Part model, mm, in its own coordinate system. Coordinates: 2 decimals unless noted, no trailing zeros. Order: outer loops, then holes, each group sorted by start corner. A loop starts at its lowest first (then second) coordinate and runs counter-clockwise, first axis right, second up.
1) Cut at B-B (x = -22.5). List the corners of the cut face in (y, z).
2) Wall check: L1, parallel to X at y = 2.5, z = 0.3; L2, parallel to Y at x = -64, z = 0.4; L3, parallel to X at y = -26, z = 0.2. Give the ranges that are in metal, low to high.
3) Pin check, flat tips, straight feed: pin 1 Ø0.9 at (x, z) = (-85, 1) entering from -Y; pin 2 Ø10 at (x, y) = (-76.5, -68.5) entering from -Z; pin 3 Ø1 at (y, z) = (41.5, 1.5) entering from -X; pin 4 Ø1.5 at (x, z) = (-86.5, 2) entering from +Y. Stop position of each tip, or through.
4) Cut at A-A (y = -1.5). List the corners of the cut face in (x, z), and give its area (3 significant figures).
5) Cut at C-C (z = 0.45). Give the number of separate pieces and of enclosed holes in the cut face, and give its area (3 significant figures).
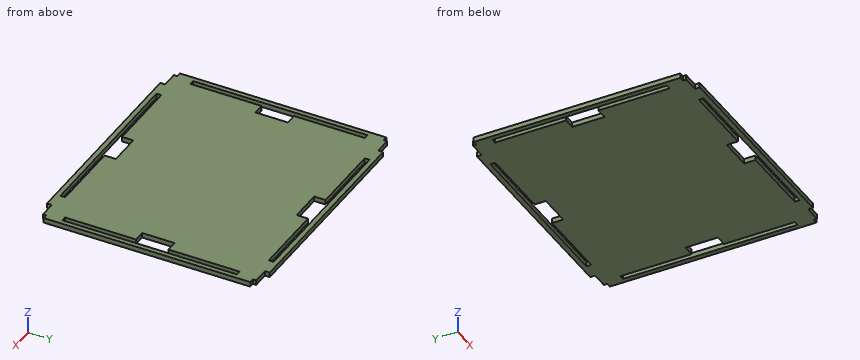
```python
from build123d import *

# Parameters (mm, degrees)
BOSS_EXTRUDE1_DEPTH = 3


with BuildPart() as part:
    # Sketch1 → Boss-Extrude1 (new body)
    with BuildSketch(Plane.XY):
        Polygon((46.640816327, 44.833717619), (-83.359183673, 44.833717619), (-83.359183673, 41.833717619), (-93.359183673, 41.833717619), (-93.359183673, 39.833717619), (-96.359183673, 39.833717619), (-96.359183673, -88.166282381), (-93.359183673, -88.166282381), (-93.359183673, -90.166282381), (-83.359183673, -90.166282381), (-83.359183673, -93.166282381), (46.640816327, -93.166282381), (46.640816327, -90.166282381), (56.640816327, -90.166282381), (56.640816327, -88.166282381), (59.640816327, -88.166282381), (59.640816327, 39.833717619), (56.640816327, 39.833717619), (56.640816327, 41.833717619), (46.640816327, 41.833717619), align=None)
        Polygon((-8.359183673, -80.166282381), (-8.359183673, -87.166282381), (36.640816327, -87.166282381), (36.640816327, -90.166282381), (-73.359183673, -90.166282381), (-73.359183673, -87.166282381), (-28.359183673, -87.166282381), (-28.359183673, -80.166282381), align=None, mode=Mode.SUBTRACT)
        Polygon((-93.359183673, -78.166282381), (-93.359183673, 29.833717619), (-90.359183673, 29.833717619), (-90.359183673, -14.166282381), (-83.359183673, -14.166282381), (-83.359183673, -34.166282381), (-90.359183673, -34.166282381), (-90.359183673, -78.166282381), align=None, mode=Mode.SUBTRACT)
        Polygon((-73.359183673, 38.833717619), (-73.359183673, 41.833717619), (36.640816327, 41.833717619), (36.640816327, 38.833717619), (-8.359183673, 38.833717619), (-8.359183673, 31.833717619), (-28.359183673, 31.833717619), (-28.359183673, 38.833717619), align=None, mode=Mode.SUBTRACT)
        Polygon((46.640816327, -34.166282381), (46.640816327, -14.166282381), (53.640816327, -14.166282381), (53.640816327, 29.833717619), (56.640816327, 29.833717619), (56.640816327, -78.166282381), (53.640816327, -78.166282381), (53.640816327, -34.166282381), align=None, mode=Mode.SUBTRACT)
    extrude(amount=BOSS_EXTRUDE1_DEPTH)


solid = part.part
```
Geometry check:
1. outline: (-93.17, 0) - (-90.17, 0) - (-90.17, 3) - (-93.17, 3) - close; (-80.17, 0) - (31.83, 0) - (31.83, 3) - (-80.17, 3) - close; (41.83, 0) - (44.83, 0) - (44.83, 3) - (41.83, 3) - close
2. L1: x = -96.36 to -93.36, -90.36 to 53.64, 56.64 to 59.64
2. L2: y = -93.17 to -90.17, -87.17 to 38.83, 41.83 to 44.83
2. L3: x = -96.36 to -93.36, -83.36 to 46.64, 56.64 to 59.64
3. pin 1: stops at y = -90.17
3. pin 2: stops at z = 0
3. pin 3: stops at x = -93.36
3. pin 4: stops at y = 41.83
4. outline: (-96.36, 0) - (-93.36, 0) - (-93.36, 3) - (-96.36, 3) - close; (-90.36, 0) - (53.64, 0) - (53.64, 3) - (-90.36, 3) - close; (56.64, 0) - (59.64, 0) - (59.64, 3) - (56.64, 3) - close
4. area: 450 mm2
5. separate pieces: 1
5. enclosed holes: 4
5. area: 19,500 mm2
